Could you check a few things on this drawing? It's one solid part, dimensions in mm from its lowest x, y, z. Give positions to 0.01 mm unless a question says otherwise; leave off trailing zeros. Order: outer loops, then holes, each group sorted by start corner. A loop starts at its lowest first (then second) coordinate and runs counter-clockwise, first axis right, second up. Notation, with made-up numbers: (31.25, 43) - (82.25, 43) arc R16 cw to (82.25, 69) - close; hole circle Ø11 at (7, -4). An arc over 180 degrees is marked (long way). Put each result on its own line as item: value.
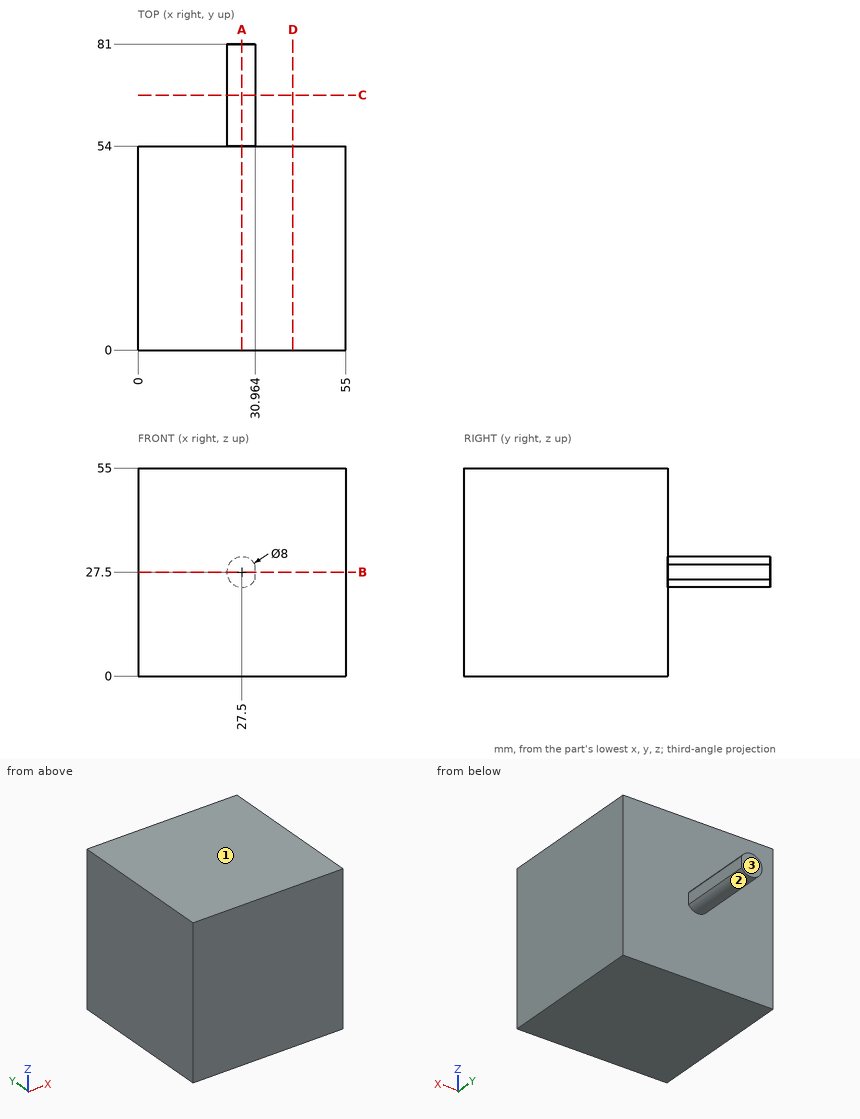
1) We'd pull the mould along Z, two halves only. Please class the marked faces 1, 2 and 3: pulls with the +Z half, pulls with the -Z half, needs draft (parallel to the pull), parting line crosses it, or undercut.
Filled in:
face 1: pulls with the +Z half
face 2: parting line crosses it
face 3: needs draft
2) If I drill on line 1 (Y direction, x = 18.5, z = 39); line 2 (X direction, y = 63, z = 28.5); line 3 (Z direction, x = 24, y = 74.5), over which ranges is the centre line in solid material (lowest first)? Write a range as [from, to].
Filled in:
line 1: y = [0, 54]
line 2: x = [23.63, 30.96]
line 3: z = [25.56, 29.44]
3) Suppose I cut it at B-B, the plane z = 27.5. List the corners of the cut face in (x, y) for me, and give its area (3 significant figures).
Filled in:
outline: (0, 0) - (55, 0) - (55, 54) - (30.96, 54) - (30.96, 81) - (23.5, 81) - (23.5, 54) - (0, 54) - close
area: 3,170 mm^2
4) I'm going to push flat-ended pins straight in: pin 1 (2 mm diameter, centred on x = 19.5, z = 23.5, fed in from -Y); pin 2 (1.2 mm diameter, centred on y = 71, z = 28, fed in from +X); pin 3 (5 mm diameter, centred on x = 17.5, z = 16.5, fed in from +Y); pin 4 (5 mm diameter, centred on x = 32, y = 62.5, fed in from +Z). Where does each tip first touch, or does it pass through?
Filled in:
pin 1: stops at y = 0
pin 2: stops at x = 30.96
pin 3: stops at y = 54
pin 4: stops at z = 30.96
5) Suppose I cut it at A-A, the plane x = 27.5. List the corners of the cut face in (y, z) for me.
Filled in:
outline: (0, 0) - (54, 0) - (54, 23.5) - (81, 23.5) - (81, 31.5) - (54, 31.5) - (54, 55) - (0, 55) - close
6) Suppose I cut it at D-D, the plane x = 41. List the corners of the cut face in (y, z) for me, and give its area (3 significant figures).
Filled in:
outline: (0, 0) - (54, 0) - (54, 55) - (0, 55) - close
area: 2,970 mm^2
7) Suppose I cut it at C-C, the plane y = 67.5. List the corners of the cut face in (x, z) for me, and give its area (3 significant figures).
Filled in:
outline: (30.96, 25.5) - (30.96, 29.5) arc R4 ccw (long way) to start
area: 48.8 mm^2
